```python
from build123d import *

# Parameters (mm, degrees)
SKETCH1_R           = 4.6609
BOSS_EXTRUDE1_DEPTH = 63.5
BOSS_EXTRUDE2_DEPTH = 6.35
FILLET1_R           = 1.27
CHAMFER1_SIZE       = 0.762
BOSS_EXTRUDE3_DEPTH = 0.254


with BuildPart() as part:
    # Sketch1 → Boss-Extrude1 (new body)
    with BuildSketch(Plane(origin=(0, 0, 0), x_dir=(1, 0, 0), z_dir=(0, 1, 0))):
        Circle(SKETCH1_R)
    extrude(amount=-BOSS_EXTRUDE1_DEPTH)

    # Sketch2 → Boss-Extrude2 (add)
    with BuildSketch(Plane(origin=(0, 0, 0), x_dir=(1, 0, 0), z_dir=(0, 1, 0))):
        Polygon((8.028921518, 0), (4.014460759, 6.95325), (-4.014460759, 6.95325), (-8.028921518, 0), (-4.014460759, -6.95325), (4.014460759, -6.95325), align=None)
    extrude(amount=BOSS_EXTRUDE2_DEPTH)

    # Fillet1
    fillet1_edges = [part.edges().sort_by_distance(p)[0] for p in [
        (6.021691139, 6.35, -3.476625),
        (6.021691139, 6.35, 3.476625),
        (0, 6.35, -6.95325),
        (-6.021691139, 6.35, -3.476625),
        (-6.021691139, 6.35, 3.476625),
        (0, 6.35, 6.95325),
    ]]
    fillet(fillet1_edges, radius=FILLET1_R)

    # Chamfer1
    chamfer1_edges = [part.edges().sort_by_distance(p)[0] for p in [
        (-4.6609, -63.5, 0),
    ]]
    chamfer(chamfer1_edges, length=CHAMFER1_SIZE)

    # Sketch3 → Boss-Extrude3 (add)
    with BuildSketch(Plane(origin=(0, 6.35, 0), x_dir=(1, 0, 0), z_dir=(0, 1, 0))):
        with BuildLine():
            Line((5.6515, -0.381), (3.2385, -0.381))
            ThreePointArc((3.2385, -0.381), (2.8575, 0), (3.2385, 0.381))
            Line((3.2385, 0.381), (5.6515, 0.381))
            ThreePointArc((5.6515, 0.381), (6.0325, 0), (5.6515, -0.381))
        make_face()
        with BuildLine():
            Line((3.155705679, 4.703842569), (1.949205679, 2.61412327))
            ThreePointArc((1.949205679, 2.61412327), (1.42875, 2.474667591), (1.289294321, 2.99512327))
            Line((1.289294321, 2.99512327), (2.495794321, 5.084842569))
            ThreePointArc((2.495794321, 5.084842569), (3.01625, 5.224298248), (3.155705679, 4.703842569))
        make_face()
        with BuildLine():
            Line((-2.495794321, 5.084842569), (-1.289294321, 2.99512327))
            ThreePointArc((-1.289294321, 2.99512327), (-1.42875, 2.474667591), (-1.949205679, 2.61412327))
            Line((-1.949205679, 2.61412327), (-3.155705679, 4.703842569))
            ThreePointArc((-3.155705679, 4.703842569), (-3.01625, 5.224298248), (-2.495794321, 5.084842569))
        make_face()
        with BuildLine():
            Line((-5.6515, 0.381), (-3.2385, 0.381))
            ThreePointArc((-3.2385, 0.381), (-2.8575, 0), (-3.2385, -0.381))
            Line((-3.2385, -0.381), (-5.6515, -0.381))
            ThreePointArc((-5.6515, -0.381), (-6.0325, 0), (-5.6515, 0.381))
        make_face()
        with BuildLine():
            Line((-3.155705679, -4.703842569), (-1.949205679, -2.61412327))
            ThreePointArc((-1.949205679, -2.61412327), (-1.42875, -2.474667591), (-1.289294321, -2.99512327))
            Line((-1.289294321, -2.99512327), (-2.495794321, -5.084842569))
            ThreePointArc((-2.495794321, -5.084842569), (-3.01625, -5.224298248), (-3.155705679, -4.703842569))
        make_face()
        with BuildLine():
            Line((2.495794321, -5.084842569), (1.289294321, -2.99512327))
            ThreePointArc((1.289294321, -2.99512327), (1.42875, -2.474667591), (1.949205679, -2.61412327))
            Line((1.949205679, -2.61412327), (3.155705679, -4.703842569))
            ThreePointArc((3.155705679, -4.703842569), (3.01625, -5.224298248), (2.495794321, -5.084842569))
        make_face()
    extrude(amount=BOSS_EXTRUDE3_DEPTH)


solid = part.part
```
Verification items for the finished model (mm, model axes). A direction names the side the tool comes from. Round coordinates to 2 decimals unless told otherwise and drop trailing zeros. Order: outer loops, then holes, each group sorted by start corner. A loop starts at its lowest first (then second) coordinate and runs counter-clockwise, first axis right, second up. Notation, with made-up numbers: (0.25, -38.75) -> (25.25, -38.75) arc R7 ccw to (25.25, -27.75) -> close; hole circle Ø6 at (17, 40.5). An arc over 180 degrees is marked (long way). Put each result on its own line as item: value. Start each with the question number.
(1) Tool access check on faces 4 (the face through (4.446, -30.93, -1.4)), 5 (the face through (-5.99, 2.5, -3.53)). Record the directions out of +Z, -Z, +X, -X, +Y, -Y that give a thin tool (end or side, any length) a straight path to the whole face; none if there is none.
(2) Material ranges on line 1 along Z through (x, y) = (0, -61); line 2 along Y through (x, z) = (-1, -5.75); line 3 along Y through (x, z) = (-2.5, -1), recorded low to high.
(3) Section check A-A (x = 0). Enter the section's corners in (y, z).
(4) Section check B-B (y = -17.5). Enter the section's corners in (x, z), then the cut area to 3 significant figures.
(5) Draft check along X on faces 1 (the face through (-6.05, 2.5, 3.43)), 2 (the face through (5.736, 5.968, 3.247)), 3 (the face through (0, 6.35, 0)). Enter one of: +X half, -X half, draft (parallel to the pull), parting line (faces both ways), or undercut.
(6) Depth check by flat-ended pin: pin 1 Ø8 at (x, y) = (-5.5, -53.5) entering from +Z; pin 2 Ø6 at (y, z) = (-6, -0.5) entering from -X; pin 3 Ø3 at (y, z) = (-42.5, -3.5) entering from -X. Enter the tip coordinate at first touch or a pass-through.
Completed:
1. face 4: -Y
1. face 5: -Z, -X, +Y, -Y
2. line 1: z = -4.66 to 4.66
2. line 2: y = 0 to 6.35
2. line 3: y = -63.5 to 6.35
3. outline: (-63.5, -3.9) -> (-62.74, -4.66) -> (0, -4.66) -> (0, -6.95) -> (5.08, -6.95) arc R1.27 ccw to (6.35, -5.68) -> (6.35, 5.68) arc R1.27 ccw to (5.08, 6.95) -> (0, 6.95) -> (0, 4.66) -> (-62.74, 4.66) -> (-63.5, 3.9) -> close
4. outline: circle Ø9.32 at (0, 0)
4. area: 68.2 mm2
5. face 1: -X half
5. face 2: +X half
5. face 3: undercut
6. pin 1: stops at z = 4.41
6. pin 2: stops at x = -4.66
6. pin 3: stops at x = -4.21
